Geometry: final body of the model. Coordinates: model frame, mm. Face numbers are marked on the shaded views. A direction names the side the tool comes from. Give positions to 0.01 mm unless a question says otherwise; leave off trailing zeros. Write each loop counter-clockwise with the first axis right and the second up, starting at its lowest first coordinate (ties: lowest second). Pieces come first, ordered by that corner, then holes. Notation, with made-up numbers: (66, -30) - (89, -30) arc R13 ccw to (89, -8) - close; hole circle Ø7 at (78.25, -12). An arc over 180 degrees is marked (long way). One line per question, with ' | ' between items. Start each with the question number.
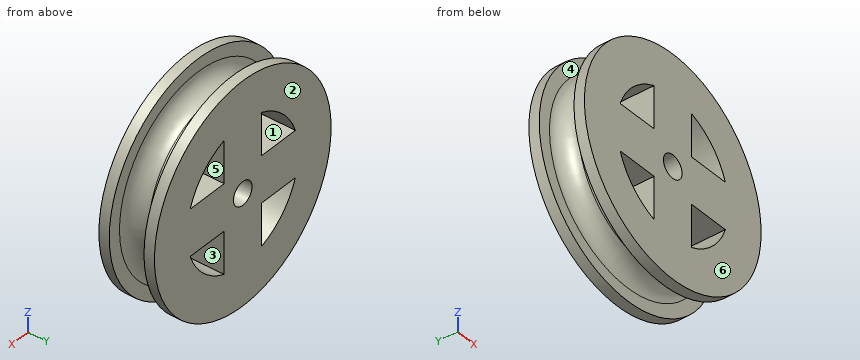
```python
from build123d import *

# Parameters (mm, degrees)
F0_R     = 23.75
F0_W     = 10
F0_H     = 10
F3_DEPTH = 6
F5_R     = 2.5
F6_DEPTH = 12.5


with BuildPart() as f3:
    # F0 (on Front) → F3 (new body, symmetric)
    with BuildSketch(Plane.XZ):
        Circle(F0_R)
        with BuildLine():
            ThreePointArc((14.1421356237, 5), (14.7839783948, 2.5365296809), (15, 0))
            ThreePointArc((15, 0), (14.7839783948, -2.5365296809), (14.1421356237, -5))
            ThreePointArc((14.1421356237, -5), (10.6066017178, -10.6066017178), (5, -14.1421356237))
            ThreePointArc((5, -14.1421356237), (0, -15), (-5, -14.1421356237))
            ThreePointArc((-5, -14.1421356237), (-10.6066017178, -10.6066017178), (-14.1421356237, -5))
            ThreePointArc((-14.1421356237, -5), (-15, 0), (-14.1421356237, 5))
            ThreePointArc((-14.1421356237, 5), (-10.6066017178, 10.6066017178), (-5, 14.1421356237))
            ThreePointArc((-5, 14.1421356237), (0, 15), (5, 14.1421356237))
            ThreePointArc((5, 14.1421356237), (10.6066017178, 10.6066017178), (14.1421356237, 5))
        make_face(mode=Mode.SUBTRACT)
        with BuildLine():
            Line((5, 5), (5, 14.1421356237))
            ThreePointArc((5, 14.1421356237), (0, 15), (-5, 14.1421356237))
            Line((-5, 14.1421356237), (-5, 5))
            Line((-5, 5), (5, 5))
        make_face()
        with BuildLine():
            ThreePointArc((14.1421356237, -5), (14.7839783948, -2.5365296809), (15, 0))
            ThreePointArc((15, 0), (14.7839783948, 2.5365296809), (14.1421356237, 5))
            Line((14.1421356237, 5), (5, 5))
            Line((5, 5), (5, -5))
            Line((5, -5), (14.1421356237, -5))
        make_face()
        Rectangle(F0_W, F0_H)
        with BuildLine():
            Line((-5, -5), (-5, 5))
            Line((-5, 5), (-14.1421356237, 5))
            ThreePointArc((-14.1421356237, 5), (-15, 0), (-14.1421356237, -5))
            Line((-14.1421356237, -5), (-5, -5))
        make_face()
        with BuildLine():
            ThreePointArc((-5, -14.1421356237), (0, -15), (5, -14.1421356237))
            Line((5, -14.1421356237), (5, -5))
            Line((5, -5), (-5, -5))
            Line((-5, -5), (-5, -14.1421356237))
        make_face()
    extrude(amount=F3_DEPTH, both=True)

    # F1 (on Right) → F4 (revolve, cut)
    with BuildSketch(Plane.YZ):
        with BuildLine():
            Line((3.75, 21), (3.75, 25))
            Line((3.75, 25), (-3.75, 25))
            Line((-3.75, 25), (-3.75, 21))
            ThreePointArc((-3.75, 21), (-2.7248737342, 18.5251262658), (-0.25, 17.5))
            Line((-0.25, 17.5), (0.25, 17.5))
            ThreePointArc((0.25, 17.5), (2.7248737342, 18.5251262658), (3.75, 21))
        make_face()
    revolve(axis=Axis((0, -2.0112972707, 0), (0, -1, 0)), mode=Mode.SUBTRACT)

    # F5 (on Front) → F6 (cut, symmetric)
    with BuildSketch(Plane.XZ):
        Circle(F5_R)
    extrude(amount=F6_DEPTH, both=True, mode=Mode.SUBTRACT)


solid = f3.part
```
1) Reachability of the marked faces 4, 5 and 6 from +Z, -Z, +X, -X, +Y, -Y: full face, straight path, thin tool, end or side. Return the list, or none.
2) Section B-B, the plane x = 0. Output: boundary loops of the cut face in (y, z), plus the area to 3 significant figures.
3) Section A-A, the plane z = 0. Output: boundary loops of the cut face in (x, y).
4) Line query: L1, parallel to X at y = -5, z = 9; L2, parallel to X at y = 1.75, z = -10.5. Output: solid intervals per line, ascending.
5) First-contact query: pin 1 Ø4.5 at (y, z) = (-2.5, -11) entering from -X; pin 2 Ø4.5 at (y, z) = (-1, 9) entering from +X; pin 3 Ø1 at (x, y) = (-7.5, -1) entering from +Z. Flat tips, straight axial feed; report the tip coordinate or a pass-through.
6) Section C-C, the plane y = 1.25. Output: boundary loops of the cut face in (x, z).
7) Pull-direction query (X, two-part tool) for the marked faces 1, 2 and 3; classes: +X half, -X half, draft (parallel to the pull), parting line (faces both ways), or undercut.
8) Section D-D, the plane x = -10. Give the number of separate pieces and of enclosed holes in the cut face, plus the area to 3 significant figures.
Answer key:
1) face 4: none | face 5: +Y, -Y | face 6: +Z, -Z, +X, -X, -Y
2) outline: (-6, -23.75) - (-3.75, -23.75) - (-3.75, -21) arc R3.5 cw to (-0.25, -17.5) - (0.25, -17.5) arc R3.5 cw to (3.75, -21) - (3.75, -23.75) - (6, -23.75) - (6, -2.5) - (-6, -2.5) - close; (-6, 2.5) - (6, 2.5) - (6, 23.75) - (3.75, 23.75) - (3.75, 21) arc R3.5 cw to (0.25, 17.5) - (-0.25, 17.5) arc R3.5 cw to (-3.75, 21) - (-3.75, 23.75) - (-6, 23.75) - close | area: 427 mm^2
3) outline: (-23.75, -6) - (-2.5, -6) - (-2.5, 6) - (-23.75, 6) - (-23.75, 3.75) - (-21, 3.75) arc R3.5 cw to (-17.5, 0.25) - (-17.5, -0.25) arc R3.5 cw to (-21, -3.75) - (-23.75, -3.75) - close; (2.5, -6) - (23.75, -6) - (23.75, -3.75) - (21, -3.75) arc R3.5 cw to (17.5, -0.25) - (17.5, 0.25) arc R3.5 cw to (21, 3.75) - (23.75, 3.75) - (23.75, 6) - (2.5, 6) - close
4) L1: -21.98 to -12, -5 to 5, 12 to 21.98 | L2: -14.42 to -10.71, -5 to 5, 10.71 to 14.42
5) pin 1: x = -21.93 | pin 2: x = 17.12 | pin 3: z = 16.17
6) outline: circle Ø35.29 at (0, 0); hole (-14.14, -5) arc R15 ccw to (-5, -14.14) - (-5, -5) - close; hole (-14.14, 5) - (-5, 5) - (-5, 14.14) arc R15 ccw to start; hole circle Ø5 at (0, 0); hole (5, -14.14) arc R15 ccw to (14.14, -5) - (5, -5) - close; hole (5, 5) - (14.14, 5) arc R15 ccw to (5, 14.14) - close
7) face 1: undercut | face 2: draft | face 3: undercut
8) separate pieces: 3 | enclosed holes: 0 | area: 274 mm^2
